```python
from build123d import *

# Parameters (mm, degrees)
SKETCH_1_W          = 26
SKETCH_1_H          = 31
EXTRUDE_1_DEPTH     = 1.5
EXTRUDE_2_DEPTH     = 1.5
SKETCH_3_R          = 4
SKETCH_3_R_2        = 1.55
CUT_EXTRUDE_1_DEPTH = 1000
FILLET_1_R          = 1.5
SKETCH_4_R          = 5
SKETCH_4_R_2        = 1.75
CUT_EXTRUDE_2_DEPTH = 100


with BuildPart() as part:
    # 草图1 → 凸台-拉伸1 (new body)
    with BuildSketch(Plane.XY):
        Rectangle(SKETCH_1_W, SKETCH_1_H)
    extrude(amount=EXTRUDE_1_DEPTH)

    # 草图2 → 凸台-拉伸2 (add)
    with BuildSketch(Plane.XZ.offset(15.5)):
        with BuildLine():
            Line((-13, 0), (13, 0))
            Line((13, 0), (13, 20))
            ThreePointArc((13, 20), (0, 33), (-13, 20))
            Line((-13, 20), (-13, 0))
        make_face()
    extrude(amount=-EXTRUDE_2_DEPTH)

    # 草图3 → 切除-拉伸1 (cut)
    with BuildSketch(Plane.XZ.offset(15.5)):
        with Locations(Location((0, 20, 0), (0, 0, 270))):
            Circle(SKETCH_3_R)
        with Locations(Location((8.5, 20, 0), (0, 0, 270))):
            Circle(SKETCH_3_R_2)
        with Locations(Location((-8.5, 20, 0), (0, 0, 270))):
            Circle(SKETCH_3_R_2)
    extrude(amount=-CUT_EXTRUDE_1_DEPTH, mode=Mode.SUBTRACT)

    # 圆角1
    fillet_1_edges = [part.edges().sort_by_distance(p)[0] for p in [
        (-13, 15.5, 0.75),
        (13, 15.5, 0.75),
    ]]
    fillet(fillet_1_edges, radius=FILLET_1_R)

    # 草图4 → 切除-拉伸2 (cut)
    with BuildSketch(Plane.XY.offset(1.5)):
        with Locations((0, 0.5)):
            Circle(SKETCH_4_R)
        with Locations((-8, 7.5)):
            Circle(SKETCH_4_R_2)
        with Locations((8, 7.5)):
            Circle(SKETCH_4_R_2)
        with Locations((-8, -6.5)):
            Circle(SKETCH_4_R_2)
        with Locations((8, -6.5)):
            Circle(SKETCH_4_R_2)
    extrude(amount=-CUT_EXTRUDE_2_DEPTH, mode=Mode.SUBTRACT)


solid = part.part
```
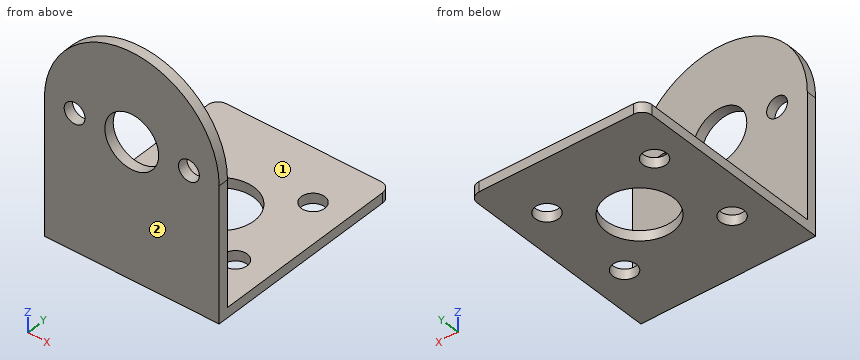
Geometry check sheet. Reference: the model listing, model coordinates, mm. Face numbers are marked on the shaded views. A direction names the side the tool comes from. Coordinates: 2 decimals unless noted, no trailing zeros. Loops run counter-clockwise (first coordinate to the right, second up) from the corner with the lowest first, then second, coordinate; pieces in that order, holes last. Notation, with made-up numbers: (-13, 59) -> (19, 59) arc R21 cw to (19, 94) -> close; hole circle Ø8 at (-31, 73). An arc over 180 degrees is marked (long way). Put each result on its own line as item: value.
1) Cross-section at C-C on x = 8. Record the boundary of the cut face in (y, z).
Result set:
outline: (-15.5, 0) -> (-8.25, 0) -> (-8.25, 1.5) -> (-14, 1.5) -> (-14, 18.53) -> (-15.5, 18.53) -> close; (-15.5, 21.47) -> (-14, 21.47) -> (-14, 30.25) -> (-15.5, 30.25) -> close; (-4.75, 0) -> (5.75, 0) -> (5.75, 1.5) -> (-4.75, 1.5) -> close; (9.25, 0) -> (15.5, 0) -> (15.5, 1.5) -> (9.25, 1.5) -> close
2) Tool access check on the marked faces 1 and 2. Record the directions out of +Z, -Z, +X, -X, +Y, -Y that give a thin tool (end or side, any length) a straight path to the whole face; none if there is none.
Result set:
face 1: +Z, +X, -X, +Y
face 2: +Z, -Z, +X, -X, -Y
3) Cross-section at D-D on y = 1.5. Record the boundary of the cut face in (x, z).
Result set:
outline: (-13, 0) -> (-4.9, 0) -> (-4.9, 1.5) -> (-13, 1.5) -> close; (4.9, 0) -> (13, 0) -> (13, 1.5) -> (4.9, 1.5) -> close
4) Cross-section at B-B on y = 7.5. Record the boundary of the cut face in (x, z), plus the area to 3 significant figures.
Result set:
outline: (-13, 0) -> (-9.75, 0) -> (-9.75, 1.5) -> (-13, 1.5) -> close; (-6.25, 0) -> (6.25, 0) -> (6.25, 1.5) -> (-6.25, 1.5) -> close; (9.75, 0) -> (13, 0) -> (13, 1.5) -> (9.75, 1.5) -> close
area: 28.5 mm^2
5) Gauge pin test, flat ends, axial feed: pin 1 Ø12 at (x, z) = (9, 17.5) entering from +Y; pin 2 Ø1.5 at (x, y) = (6.5, 4) entering from +Z. Record the tip position at first contact, or that the pin passes through.
Result set:
pin 1: stops at y = -14
pin 2: stops at z = 1.5
6) Cross-section at A-A on x = 0. Record the boundary of the cut face in (y, z).
Result set:
outline: (-15.5, 0) -> (-4.5, 0) -> (-4.5, 1.5) -> (-14, 1.5) -> (-14, 16) -> (-15.5, 16) -> close; (-15.5, 24) -> (-14, 24) -> (-14, 33) -> (-15.5, 33) -> close; (5.5, 0) -> (15.5, 0) -> (15.5, 1.5) -> (5.5, 1.5) -> close
7) Thickness scan on line 1 (Y direction, x = -8, z = 0.9); line 2 (X direction, y = 6, z = 1); line 3 (Y direction, x = -2.25, z = 2.5). Record the ranges inside material, lowest first.
Result set:
line 1: y = -15.5 to -8.25, -4.75 to 5.75, 9.25 to 15.5
line 2: x = -13 to -8.9, -7.1 to 7.1, 8.9 to 13
line 3: y = -15.5 to -14
